```python
from build123d import *

# Parameters (mm, degrees)
SKETCH003_R     = 1.5
PAD010_DEPTH    = 8
SKETCH017_R     = 1.5
PAD009_DEPTH    = 8
SKETCH016_R     = 2.5
POCKET001_DEPTH = 15
CHAMFER005_SIZE = 0.5


with BuildPart() as pad010:
    # Sketch003 → Pad010 (new body)
    with BuildSketch(Plane(origin=(7, 0, 3.5), x_dir=(0, 1, 0), z_dir=(1, 0, 0))):
        Circle(SKETCH003_R)
    extrude(amount=-PAD010_DEPTH)


with BuildPart() as pad009:
    # Sketch017 → Pad009 (new body)
    with BuildSketch(Plane(origin=(0, -7, 3.5), x_dir=(1, 0, 0), z_dir=(0, -1, 0))):
        Circle(SKETCH017_R)
    extrude(amount=-PAD009_DEPTH)


with BuildPart() as chamfer005:
    # Sketch015 → Revolution (revolve)
    with BuildSketch(Plane.XZ):
        Polygon((0, 0), (6.5, 0), (6.5, 7), (4.7, 7), (4.7, 14), (6.5, 14), (6.5, 15), (0, 15), align=None)
    revolve(axis=Axis((0, 0, 0), (0, 0, 1)))

    # Sketch016 (on Face7 of Revolution) → Pocket001 (cut)
    with BuildSketch(Plane(origin=(0, 0, 15), x_dir=(-1, 0, 0), z_dir=(0, 0, 1))):
        Circle(SKETCH016_R)
    extrude(amount=-POCKET001_DEPTH, mode=Mode.SUBTRACT)

    # Cut013: cut Pad009
    add(pad009.part, mode=Mode.SUBTRACT)

    # Cut014: cut Pad010
    add(pad010.part, mode=Mode.SUBTRACT)

    # Chamfer005
    chamfer005_edges = [chamfer005.edges().sort_by_distance(p)[0] for p in [
        (-4e-06, -6.499997, 4.999986),
        (-4e-06, -6.499997, 2.000014),
        (6.412872, 1.060693, 4.560627),
        (6.412872, 1.060693, 2.439373),
        (6.412872, -1.060693, 2.439373),
        (6.412872, -1.060693, 4.560627),
    ]]
    chamfer(chamfer005_edges, length=CHAMFER005_SIZE)


solid = chamfer005.part
```
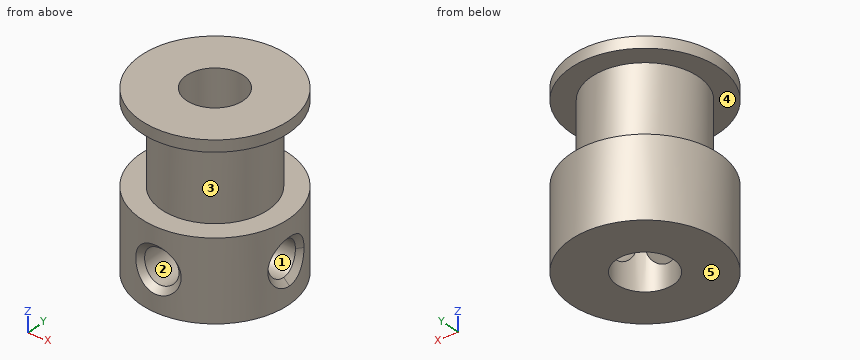
The model under review builds one solid part; all positions refer to its coordinate system, in mm. Face numbers are marked on the shaded views. A direction names the side the tool comes from. Give positions to 0.01 mm unless a question says otherwise; leave off trailing zeros. Write each loop counter-clockwise with the first axis right and the second up, starting at its lowest first coordinate (ties: lowest second). Pieces come first, ordered by that corner, then holes. Notation, with made-up numbers: (-30.75, -21) - (17.25, -21) arc R15 ccw to (17.25, -3) - close; hole circle Ø10 at (9, -17). An arc over 180 degrees is marked (long way). Answer in a Markdown table with one row per item. Add a question column.
1. Insertion check: P1, Ø3, axis at y = 4.5, z = 9.5, coming from the -X side; P2, Ø5, axis at x = 4, z = 12, coming from the -Y side; P3, Ø2.5, axis at y = 0, z = 3.5, coming from the +X side. Each pin has a flat end and moves straight along its axis. Give the tip position at first contact, or say it passes through.
2. We need section B-B on z = 12.5. Write out the cut boundary in (x, y), then the cut area to 3 significant figures.
3. Tool access review of the marked faces 4 and 5: name each direction out of +Z, -Z, +X, -X, +Y, -Y from which nothing blocks a thin tool from reaching the whole face with its end or side.
4. We need section A-A on x = 4. Write out the cut boundary in (y, z), then the cut area to 3 significant figures.
5. Draft analysis for pull direction X (two halves, no side actions). For the marked faces 1, 2 and 3, state which applies: +X half, -X half, draft (parallel to the pull), parting line (faces both ways), or undercut.
6. Wall thickness on line 1 along Y through (x, z) = (0, 8.75); line 2 along Z through (x, y) = (4.4, 0); line 3 along Z through (x, y) = (2.5, -5.75): over which ranges is each line inside the solid? List them lowest first. Write a range as [from, to].
7. We need section C-C on x = -5. Write out the cut boundary in (y, z).
8. We need section D-D on y = 3.25. Write out the cut boundary in (x, z), then the cut area to 3 significant figures.
Ans:
| question | item | result |
|---|---|---|
| 1 | P1 | stops at x = -3.62 |
| 1 | P2 | stops at y = -6 |
| 1 | P3 | stops at x = -2.17 |
| 2 | outline | circle Ø9.4 at (0, 0); hole circle Ø5 at (0, 0) |
| 2 | area | 49.8 mm^2 |
| 3 | face 4 | none |
| 3 | face 5 | -Z, +X, -X, +Y, -Y |
| 4 | outline | (-5.12, 0) - (5.12, 0) - (5.12, 7) - (2.47, 7) - (2.47, 14) - (5.12, 14) - (5.12, 15) - (-5.12, 15) - (-5.12, 14) - (-2.47, 14) - (-2.47, 7) - (-5.12, 7) - close; hole circle Ø3 at (0, 3.5) |
| 4 | area | 109 mm^2 |
| 5 | face 1 | draft |
| 5 | face 2 | undercut |
| 5 | face 3 | parting line |
| 6 | line 1 | y = [-4.7, -2.5], [2.5, 4.7] |
| 6 | line 2 | z = [0, 2], [5, 15] |
| 6 | line 3 | z = [0, 7], [14, 15] |
| 7 | outline | (-4.15, 0) - (4.15, 0) - (4.15, 7) - (-4.15, 7) - close; (-4.15, 14) - (4.15, 14) - (4.15, 15) - (-4.15, 15) - close |
| 8 | outline | (-5.63, 0) - (5.63, 0) - (5.63, 7) - (3.4, 7) - (3.4, 14) - (5.63, 14) - (5.63, 15) - (-5.63, 15) - (-5.63, 14) - (-3.4, 14) - (-3.4, 7) - (-5.63, 7) - close |
| 8 | area | 138 mm^2 |
